Could you check a few things on this drawing? It's one solid part, dimensions in mm from its lowest x, y, z. A direction names the side the tool comes from. Round coordinates to 2 decimals unless told otherwise and drop trailing zeros. Write each loop counter-clockwise with the first axis right and the second up, starting at its lowest first coordinate (ties: lowest second). Pieces come first, ordered by that corner, then holes. Notation, with made-up numbers: M 34,6 L 73,6 A26 cw 73,30 Z; hole C -7,28.25 d9. An arc over 180 degrees is marked long. One line per item, written item: value. Start each with the question number.
(1) I want a section at D-D on x = 19.5. Count the separate pieces of the cut face and the enclosed holes in it, and give its area (3 significant figures).
(2) Which directions (+Z, -Z, +X, -X, +Y, -Y) give clear straight access to the entire face, cutting with the end or side of a thin tool? Please do the marked faces 1 and 2.
(3) Thinking about a two-plate mould opening in X: for the marked faces 3, 4, 5 and 6, which applies, released by +X, released by -X, zero draft, split by the parting line, or undercut?
(4) If I drill on L1, parallel to X at y = 31, z = 3; L2, parallel to X at y = 14, z = 10; L3, parallel to Y at x = 16, z = 3.25, over which ranges is the centre line in solid material (lowest first)?
(5) I want a section at C-C on y = 24. Please give me the cut outline in (x, z), and give its area (3 significant figures).
(6) I want a section at A-A on x = 10. Please give me the cut outline in (y, z).
(7) I'm going to push flat-ended pins straight in: pin 1 Ø3 at (x, z) = (3, 3) entering from -Y; pin 2 Ø4 at (x, y) = (12.5, 17) entering from -Z; pin 3 Ø5 at (y, z) = (22, 7) entering from -X; pin 4 Ø1.6 at (x, z) = (20, 17) entering from -Y. Where does each tip first touch, or does it pass through?
(8) I want a section at B-B on z = 10. Please give me the cut outline in (x, y), and give its area (3 significant figures).
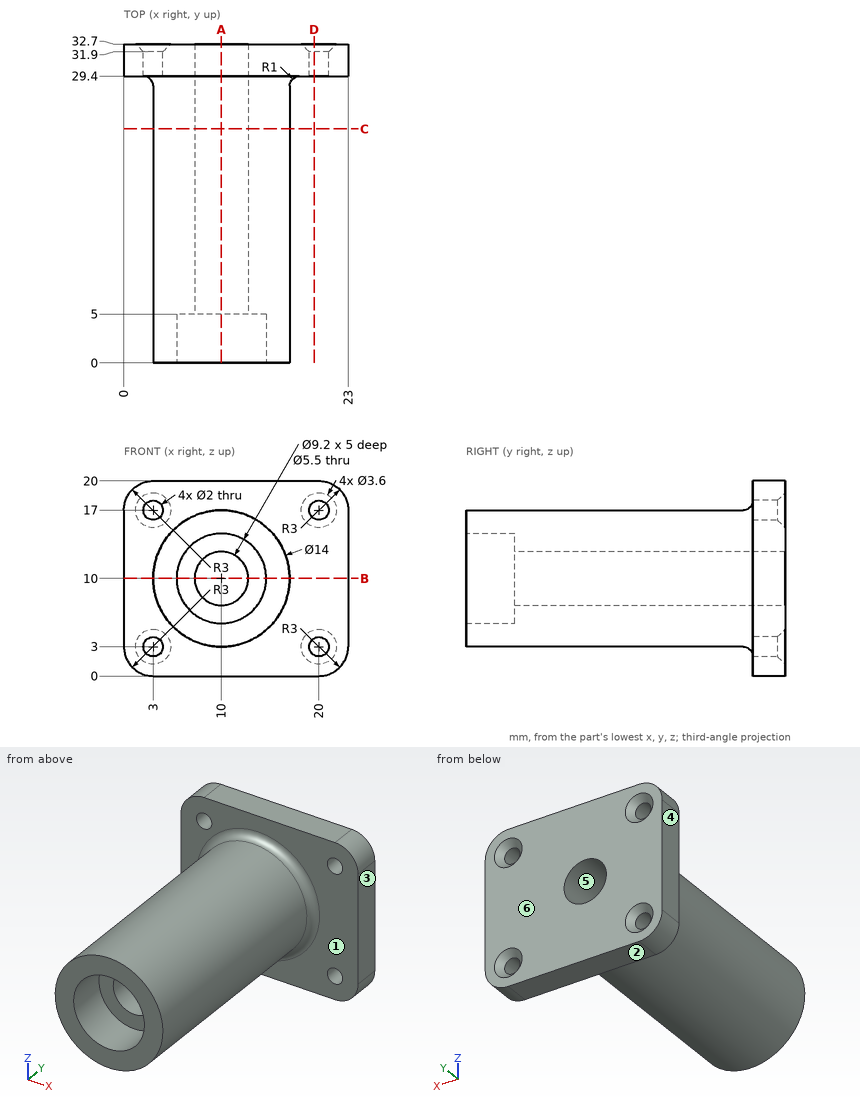
Found:
1. separate pieces: 3
1. enclosed holes: 0
1. area: 53.2 mm²
2. face 1: -Y
2. face 2: -Z, +X, -X, +Y, -Y
3. face 3: released by +X
3. face 4: released by -X
3. face 5: undercut
3. face 6: zero draft
4. L1: x = 0 to 2, 4 to 19, 21 to 23
4. L2: x = 3 to 7.25, 12.75 to 17
4. L3: y = 29.4 to 32.7
5. outline: C 10,10 d14; hole C 10,10 d5.5
5. area: 130 mm²
6. outline: M 0,3 L 28.4,3 A1 cw 29.4,2 L 29.4,0 L 32.7,0 L 32.7,7.25 L 5,7.25 L 5,5.4 L 0,5.4 Z; M 0,14.6 L 5,14.6 L 5,12.75 L 32.7,12.75 L 32.7,20 L 29.4,20 L 29.4,18 A1 cw 28.4,17 L 0,17 Z
7. pin 1: stops at y = 29.4
7. pin 2: stops at z = 3.02
7. pin 3: stops at x = 3.02
7. pin 4: passes through
8. outline: M 0,29.4 L 2,29.4 A1 cw 3,28.4 L 3,0 L 5.4,0 L 5.4,5 L 7.25,5 L 7.25,32.7 L 0,32.7 Z; M 12.75,5 L 14.6,5 L 14.6,0 L 17,0 L 17,28.4 A1 cw 18,29.4 L 23,29.4 L 23,32.7 L 12.75,32.7 Z
8. area: 290 mm²
